Verification items for the finished model (mm, model axes). Coordinates: 2 decimals unless noted, no trailing zeros. Loops run counter-clockwise (first coordinate to the right, second up) from the corner with the lowest first, then second, coordinate; pieces in that order, holes last. Notation, with made-up numbers: (-25, -12) - (-14, -12) arc R20 ccw to (-14, -1) - close; hole circle Ø8 at (17.25, 2.5). An arc over 180 degrees is marked (long way). Answer as CSV lines item,"result". Start each with the question number.
1. Release check for a two-part mould opening along X. For faces 1 (the flat face through (0, 4, -2.5)), 2 (the flat face through (7.306, 4.19, 8.259)), 3 (the cylindrical face through (0, 4, 16)), 4 (the cylindrical face through (0, 4, 3)) record: pulls with the +X half, pulls with the -X half, needs draft (parallel to the pull), parting line crosses it, or undercut.
2. Cross-section at B-B (x = 0). Enter the section's corners in (y, z).
3. Cross-section at A-A (z = 0). Enter the section's corners in (x, y), plus the area to 3 significant figures.
4. Cross-section at D-D (x = -6.5). Enter the section's corners in (y, z), plus the area to 3 significant figures.
5. Cross-section at C-C (y = 3.5). Enter the section's corners in (x, z).
6. Material ranges on line 1 (X direction, y = 2.5, z = 0); line 2 (Z direction, x = -0.75, y = 4.5); line 3 (X direction, y = 3, z = 1.25), recorded low to high. Write a range as [from, to].
7. Gauge pin test, flat ends, axial feed: P1, Ø1, axis at y = 3, z = 3, coming from the -X side; P2, Ø3, axis at x = -7, y = 3, coming from the -Z side; P3, Ø1, axis at x = 1, y = 4, coming from the +Z side; P4, Ø1.5, axis at x = 0, z = 1, coming from the -Y side. Record the tip position at first contact, or that the pin passes through.
```python
from build123d import *

# Parameters (mm, degrees)
BOSS_EXTRUDE1_DEPTH = 8.5


with BuildPart() as part:
    # Sketch1 → Boss-Extrude1 (new body)
    with BuildSketch(Plane(origin=(0, 0, 0), x_dir=(1, 0, 0), z_dir=(0, 1, 0))):
        with BuildLine():
            Line((-9.16515139, -4), (-5.499090834, -12.4))
            ThreePointArc((-5.499090834, -12.4), (0, -16), (5.499090834, -12.4))
            Line((5.499090834, -12.4), (9.16515139, -4))
            ThreePointArc((9.16515139, -4), (0, 10), (-9.16515139, -4))
        make_face()
        with BuildLine():
            Line((1.658301541, 2.5), (-1.658301541, 2.5))
            ThreePointArc((-1.658301541, 2.5), (0, -2.999994), (1.658301541, 2.5))
        make_face(mode=Mode.SUBTRACT)
    extrude(amount=BOSS_EXTRUDE1_DEPTH)


solid = part.part
```
Values follow:
1,face 1,"undercut"
1,face 2,"pulls with the +X half"
1,face 3,"parting line crosses it"
1,face 4,"undercut"
2,outline,"(0, -10) - (8.5, -10) - (8.5, -2.5) - (0, -2.5) - close; (0, 3) - (8.5, 3) - (8.5, 16) - (0, 16) - close"
3,outline,"(-10, 0) - (-3, 0) - (-3, 8.5) - (-10, 8.5) - close; (3, 0) - (10, 0) - (10, 8.5) - (3, 8.5) - close"
3,area,"119 mm²"
4,outline,"(0, -7.6) - (8.5, -7.6) - (8.5, 10.11) - (0, 10.11) - close"
4,area,"151 mm²"
5,outline,"(-9.17, 4) arc R10 ccw (long way) to (9.17, 4) - (5.5, 12.4) arc R6 ccw to (-5.5, 12.4) - close; hole (-1.66, -2.5) - (1.66, -2.5) arc R3 ccw (long way) to start"
6,line 1,"x = [-10, -3], [3, 10]"
6,line 2,"z = [-9.97, -2.5], [2.9, 15.95]"
6,line 3,"x = [-9.92, -2.73], [2.73, 9.92]"
7,P1,"stops at x = -9.68"
7,P2,"stops at z = -8.35"
7,P3,"stops at z = 15.98"
7,P4,"passes through"
